```python
from build123d import *

# Parameters (mm, degrees)
F2_W     = 8
F2_H     = 10
F3_DEPTH = 30.001
F4_SIZE  = 1.5


with BuildPart() as f1:
    # F0 (on Front) → F1 (revolve)
    with BuildSketch(Plane.XZ):
        Polygon((7, 68.5), (0, 68.5), (0, 12.5), (30, 12.5), (30, 33), (7, 33), align=None)
    revolve(axis=Axis((33.79849, 0, 0), (1, 0, 0)))

    # F2 (on Right) → F3 (cut, through all)
    with BuildSketch(Plane.YZ):
        with Locations((0, 11)):
            Rectangle(F2_W, F2_H)
    extrude(amount=F3_DEPTH, mode=Mode.SUBTRACT)

    # F4
    f4_edges = [f1.edges().sort_by_distance(p)[0] for p in [
        (7, 0, -68.5),
        (0, 0, -68.5),
    ]]
    chamfer(f4_edges, length=F4_SIZE)


solid = f1.part
```
Input: part model. Units: mm. Frame: model coordinates. A direction names the side the tool comes from. Round coordinates to 2 decimals unless told otherwise and drop trailing zeros. Loops run counter-clockwise (first coordinate to the right, second up) from the corner with the lowest first, then second, coordinate; pieces in that order, holes last.
1) Pin query (flat end, axial travel): pin 1 (1.5 mm diameter, centred on x = 23, y = -20.5, fed in from -Z); pin 2 (4 mm diameter, centred on y = -15.5, z = -45.5, fed in from +X); pin 3 (8 mm diameter, centred on x = 13.5, y = 33, fed in from -Z). Return the tip coordinate at first contact, or that it passes through.
Ans:
pin 1: stops at z = -26.44
pin 2: stops at x = 7
pin 3: stops at z = -15.75
2) Material intervals for line 1 (Z direction, x = 9, y = 0); line 2 (Y direction, x = 12.75, z = 0); line 3 (X direction, y = -34.5, z = 17.5), sorted ascending.
Ans:
line 1: z = -33 to -12.5, 16 to 33
line 2: y = -33 to -12.5, 12.5 to 33
line 3: x = 0 to 7
3) Section query A-A on y = 0. Return the cut outline in (x, z).
Ans:
outline: (0, -67) - (1.5, -68.5) - (5.5, -68.5) - (7, -67) - (7, -33) - (30, -33) - (30, -12.5) - (0, -12.5) - close; (0, 16) - (30, 16) - (30, 33) - (7, 33) - (7, 67) - (5.5, 68.5) - (1.5, 68.5) - (0, 67) - close
4) Section query C-C on x = 24.5. Return the cut outline in (y, z).
Ans:
outline: circle Ø66 at (0, 0); hole (-4, 11.84) arc R12.5 ccw (long way) to (4, 11.84) - (4, 16) - (-4, 16) - close
5) Set-up query: faces 1 (the flat face through (7, 14, 31)), 2 (the flat face through (30, 0, -14)), 3 (the flat face through (15, 0, 16)). Return all of +Z, -Z, +X, -X, +Y, -Y with unobstructed straight access to the full face (end or side cutting, diameter ignored); none if empty.
Ans:
face 1: +X
face 2: +Z, -Z, +X, +Y, -Y
face 3: +X, -X
6) Section query B-B on z = 0. Return the cut outline in (x, y).
Ans:
outline: (0, -67) - (1.5, -68.5) - (5.5, -68.5) - (7, -67) - (7, -33) - (30, -33) - (30, -12.5) - (0, -12.5) - close; (0, 12.5) - (30, 12.5) - (30, 33) - (7, 33) - (7, 67) - (5.5, 68.5) - (1.5, 68.5) - (0, 67) - close
7) Pull-direction query (Y, two-part tool) for faces 4 (the cylindrical face through (18.3, 12.6, 30.5)), 5 (the cylindrical face through (15.21, -0.49, -12.49)), 6 (the flat face through (0, 14, -1)), 7 (the flat face through (15, -4, 14)); classes: released by +Y, released by -Y, zero draft, split by the parting line, or undercut.
Ans:
face 4: split by the parting line
face 5: undercut
face 6: zero draft
face 7: undercut
